```python
from build123d import *

# Parameters (mm, degrees)
SKETCH4_R           = 42.545
BOSS_EXTRUDE2_DEPTH = 0.254
SKETCH5_R           = 15.875
CUT_EXTRUDE5_DEPTH  = 1.254
CUT_EXTRUDE11_DEPTH = 1.254
SKETCH9_R           = 4.699
CUT_EXTRUDE12_DEPTH = 1.254


with BuildPart() as part:
    # Sketch4 → Boss-Extrude2 (new body)
    with BuildSketch(Plane.XY):
        Circle(SKETCH4_R)
    extrude(amount=BOSS_EXTRUDE2_DEPTH)

    # Sketch5 → Cut-Extrude5 (cut, through all)
    with BuildSketch(Plane.XY.offset(0.254)):
        Circle(SKETCH5_R)
    extrude(amount=-CUT_EXTRUDE5_DEPTH, mode=Mode.SUBTRACT)

    # Sketch8 → Cut-Extrude11 (cut, through all)
    with BuildSketch(Plane.XY.offset(0.254)):
        Polygon((40.379126173, 15.350943603), (39.407110255, 17.697597616), (38.233783248, 17.211589657), (39.205799167, 14.864935644), align=None)
        Polygon((-15.350943603, 40.379126173), (-17.697597616, 39.407110255), (-17.211589657, 38.233783248), (-14.864935644, 39.205799167), align=None)
        Polygon((-39.407110255, 17.697597616), (-40.379126173, 15.350943603), (-39.205799167, 14.864935644), (-38.233783248, 17.211589657), align=None)
        Polygon((-40.379126173, -15.350943603), (-39.407110255, -17.697597616), (-38.233783248, -17.211589657), (-39.205799167, -14.864935644), align=None)
        Polygon((-17.697597616, -39.407110255), (-15.350943603, -40.379126173), (-14.864935644, -39.205799167), (-17.211589657, -38.233783248), align=None)
        Polygon((15.350943603, -40.379126173), (17.697597616, -39.407110255), (17.211589657, -38.233783248), (14.864935644, -39.205799167), align=None)
        Polygon((39.407110255, -17.697597616), (40.379126173, -15.350943603), (39.205799167, -14.864935644), (38.233783248, -17.211589657), align=None)
        Polygon((17.697597616, 39.407110255), (15.350943603, 40.379126173), (14.864935644, 39.205799167), (17.211589657, 38.233783248), align=None)
    extrude(amount=-CUT_EXTRUDE11_DEPTH, mode=Mode.SUBTRACT)

    # Sketch9 → Cut-Extrude12 (cut, through all)
    with BuildSketch(Plane.XY.offset(0.254)):
        with Locations((22.225, 0)):
            Circle(SKETCH9_R)
        with Locations((36.195, 0)):
            Circle(SKETCH9_R)
        with Locations((15.715448212, -15.715448212)):
            Circle(SKETCH9_R)
        with Locations((25.593729945, -25.593729945)):
            Circle(SKETCH9_R)
        with Locations((0, -22.225)):
            Circle(SKETCH9_R)
        with Locations((0, -36.195)):
            Circle(SKETCH9_R)
        with Locations((-15.715448212, -15.715448212)):
            Circle(SKETCH9_R)
        with Locations((-25.593729945, -25.593729945)):
            Circle(SKETCH9_R)
        with Locations((-22.225, 0)):
            Circle(SKETCH9_R)
        with Locations((-36.195, 0)):
            Circle(SKETCH9_R)
        with Locations((-15.715448212, 15.715448212)):
            Circle(SKETCH9_R)
        with Locations((-25.593729945, 25.593729945)):
            Circle(SKETCH9_R)
        with Locations((0, 22.225)):
            Circle(SKETCH9_R)
        with Locations((0, 36.195)):
            Circle(SKETCH9_R)
        with Locations((15.715448212, 15.715448212)):
            Circle(SKETCH9_R)
        with Locations((25.593729945, 25.593729945)):
            Circle(SKETCH9_R)
    extrude(amount=-CUT_EXTRUDE12_DEPTH, mode=Mode.SUBTRACT)


solid = part.part
```
Read the model definition and answer for the solid it produces. Units are mm, in the model's axes. Round coordinates to 2 decimals unless told otherwise and drop trailing zeros. Write each loop counter-clockwise with the first axis right and the second up, starting at its lowest first coordinate (ties: lowest second). Pieces come first, ordered by that corner, then holes. Notation, with made-up numbers: (33.5, 29) -> (88.5, 29) arc R36 cw to (88.5, 67) -> close; hole circle Ø4 at (-38.5, 27.25). An arc over 180 degrees is marked (long way). Answer in a Markdown table with one row per item. Add a question column.
1) Find section C-C, the plane y = -33. Determine the outline of the cut face in (x, z), and give its area (3 significant figures).
2) Find section D-D, the plane x = 24. Determine the outline of the cut face in (y, z).
3) Find section A-A, the plane y = 0. Determine the outline of the cut face in (x, z) (3 decimals).
4) Consider line 1 (Y direction, x = 0, z = 0.1) (3 decimals); line 2 (Y direction, x = 12, z = 0.1); line 3 (X direction, y = 14.5, z = 0.1). Determine where each line is inside the solid, lowest interval first.
Findings below:
| question | item | result |
|---|---|---|
| 1 | outline | (-26.85, 0) -> (-3.45, 0) -> (-3.45, 0.25) -> (-26.85, 0.25) -> close; (3.45, 0) -> (26.85, 0) -> (26.85, 0.25) -> (3.45, 0.25) -> close |
| 1 | area | 11.9 mm² |
| 2 | outline | (-35.13, 0) -> (-30.01, 0) -> (-30.01, 0.25) -> (-35.13, 0.25) -> close; (-21.17, 0) -> (-4.35, 0) -> (-4.35, 0.25) -> (-21.17, 0.25) -> close; (4.35, 0) -> (21.17, 0) -> (21.17, 0.25) -> (4.35, 0.25) -> close; (30.01, 0) -> (35.13, 0) -> (35.13, 0.25) -> (30.01, 0.25) -> close |
| 3 | outline | (-42.545, 0) -> (-40.894, 0) -> (-40.894, 0.254) -> (-42.545, 0.254) -> close; (-31.496, 0) -> (-26.924, 0) -> (-26.924, 0.254) -> (-31.496, 0.254) -> close; (-17.526, 0) -> (-15.875, 0) -> (-15.875, 0.254) -> (-17.526, 0.254) -> close; (15.875, 0) -> (17.526, 0) -> (17.526, 0.254) -> (15.875, 0.254) -> close; (26.924, 0) -> (31.496, 0) -> (31.496, 0.254) -> (26.924, 0.254) -> close; (40.894, 0) -> (42.545, 0) -> (42.545, 0.254) -> (40.894, 0.254) -> close |
| 4 | line 1 | -42.545 to -40.894, -31.496 to -26.924, -17.526 to -15.875, 15.875 to 17.526, 26.924 to 31.496, 40.894 to 42.545 |
| 4 | line 2 | -40.82 to -18.59, -12.84 to -10.39, 10.39 to 12.84, 18.59 to 40.82 |
| 4 | line 3 | -40 to -20.25, -11.18 to -6.46, 6.46 to 11.18, 20.25 to 40 |
